Autodesk Fusion 360 part; units mm, degrees
sketch "Sketch1" plane through (0, 0, 0) normal (0, 1, 0) x (1, 0, 0)
  line L0 (0, 0) -> (162.5, 0)
  line L1 (162.5, 0) -> (162.5, 40)
  line L2 (162.5, 40) -> (0, 40)
  line L3 (0, 40) -> (0, 0)
  dimension "d1" = 162.5
  dimension "d2" = 40
extrude "Extrude1" add sketch "Sketch1" along normal blind 5
sketch "Sketch2" plane through (0, 5, 0) normal (0, 1, 0) x (-1, 0, 0)
  line L0 (0, -40) -> (0, 0)
  line L1 (0, 0) -> (-162.5, 0)
  line L2 (-162.5, 0) -> (-162.5, -40)
  line L3 (-162.5, -40) -> (0, -40)
  line L4 (-162.5, -40) -> (-152.5, -40)
  line L5 (-152.5, -40) -> (-152.5, 0)
  line L6 (-152.5, 0) -> (-162.5, 0)
  line L7 (-162.5, 0) -> (-162.5, -40)
  dimension "d10" = 10
extrude "Extrude2" add sketch "Sketch2" along normal blind 10 contours L1 L2 L3 L4 L5 L6 L7
sketch "Sketch3" plane through (152.5, 0, 0) normal (-1, 0, 0) x (0, 0, 1)
  line L0 (-40, 5) -> (0, 5)
  line L1 (0, 5) -> (0, 15)
  line L2 (0, 15) -> (-40, 15)
  line L3 (-40, 15) -> (-40, 5)
  line L4 (-40, 15) -> (0, 5) construction
  line L5 (-40, 5) -> (0, 15) construction
  circle A0 centre (-20, 10) radius 1.6
  circle A1 centre (-20, 10) radius 2.85
  dimension "d7" = 3.2
  dimension "d15" = 5.7
extrude "Extrude3" cut sketch "Sketch3" against normal blind 10.5 contours A0
fillet "Fillet1" radius 5 1 edges at (157.5, 15, 0)
extrude "Extrude4" cut sketch "Sketch3" along normal blind -5 and the other way blind 0 contours A1
fillet "Fillet3" radius 5 1 edges at (152.5, 5, -20)
fillet "Fillet4" radius 5 1 edges at (157.5, 15, -40)
Could you check a few things on this model? Use its own coordinates, in mm. A direction names the side the tool comes from. Coordinates: 2 decimals unless noted, no trailing zeros. Order: outer loops, then holes, each group sorted by start corner. A loop starts at its lowest first (then second) coordinate and runs counter-clockwise, first axis right, second up. Notation, with made-up numbers: (34, -33.75) - (88, -33.75) arc R28 ccw to (88, -6.75) - close; hole circle Ø6 at (-29, 72.25). An arc over 180 degrees is marked (long way). Answer in a Markdown table with one row per item. Add a question column.
(1) If we section it at B-B, the plane x = 112: Please give me the cut outline in (y, z).
(2) If we mould it in two halves opening along Z, with no side actions, what happens to faces 4 (the face through (80, 3, 0)), 5 (the face through (73, 5, -20)), 6 (the face through (157.5, 8, -20))? For each: released by +Z, released by -Z, zero draft, split by the parting line, or undercut.
(3) If we section it at A-A, the plane z = -25.5: Please give me the cut outline in (x, y) (3 decimals).
(4) I need wall thicknesses on L1, parallel to Z at x = 155.1, y = 10; L2, parallel to Y at x = 155, z = -20; L3, parallel to Y at x = 161.4, z = -20. Which ranges of each line are inside material? Lowest first, please.
(5) Will these pins go through, and if not, where does the flat tip stop? pin 1 (3.5 mm diameter, centred on y = 10, z = -20, fed in from -X); pin 2 (6 mm diameter, centred on x = 48, y = 9, fed in from +Z); pin 3 (1 mm diameter, centred on y = 10.5, z = -10.5, fed in from -X); pin 4 (1.5 mm diameter, centred on x = 109.5, z = -21.5, fed in from +Y).
(6) On a 3-axis mill with a long thin cutter (end or side, diameter ignored), from which of +Z, -Z, +X, -X, +Y, -Y can I reach the whole of each face in a straight line? I mean faces 1 (the face through (80, 0, -20)), 2 (the face through (152.5, 13, -20)), 3 (the face through (154.965, 11.926, -22.101)). Say none if no direction works.
Results are:
| question | item | result |
|---|---|---|
| 1 | outline | (0, -40) - (5, -40) - (5, 0) - (0, 0) - close |
| 2 | face 4 | released by +Z |
| 2 | face 5 | zero draft |
| 2 | face 6 | undercut |
| 3 | outline | (0, 0) - (162.5, 0) - (162.5, 15) - (152.5, 15) - (152.5, 9.975) arc R4.975 cw to (147.525, 5) - (0, 5) - close |
| 4 | L1 | z = -40 to -22.85, -17.15 to 0 |
| 4 | L2 | y = 0 to 7.15, 12.85 to 15 |
| 4 | L3 | y = 0 to 8.4, 11.6 to 15 |
| 5 | pin 1 | stops at x = 157.5 |
| 5 | pin 2 | passes through |
| 5 | pin 3 | stops at x = 152.5 |
| 5 | pin 4 | stops at y = 5 |
| 6 | face 1 | +Z, -Z, +X, -X, -Y |
| 6 | face 2 | +Z, -Z, -X, +Y |
| 6 | face 3 | -X |
